from build123d import *

# Parameters (mm, degrees)
SKETCH4_R           = 2.5
BOSS_EXTRUDE1_DEPTH = 25
SKETCH5_R           = 2.5
CUT_EXTRUDE1_DEPTH  = 55.976783394
SKETCH6_R           = 3.25
CUT_EXTRUDE2_DEPTH  = 1
SKETCH7_R           = 2.5
CUT_EXTRUDE3_DEPTH  = 46.809522816
SKETCH8_R           = 3.25
CUT_EXTRUDE4_DEPTH  = 1


with BuildPart() as part:
    # Sketch4 → Boss-Extrude1 (new body)
    with BuildSketch(Plane(origin=(0, 0, 0), x_dir=(1, 0, 0), z_dir=(0, 1, 0))):
        with BuildLine():
            Line((12.859651739, 14.301163983), (32.859651739, 14.301163983))
            Line((32.859651739, 14.301163983), (32.859651739, 19.301163983))
            Line((32.859651739, 19.301163983), (12.859651739, 19.301163983))
            Line((12.859651739, 19.301163983), (12.859651739, 22.501163983))
            Line((12.859651739, 22.501163983), (3.559651739, 22.501163983))
            ThreePointArc((3.559651739, 22.501163983), (-3.511416073, 19.572231795), (-6.440348261, 12.501163983))
            Line((-6.440348261, 12.501163983), (-6.440348261, 3.001163983))
            Line((-6.440348261, 3.001163983), (-3.240348261, 3.001163983))
            Line((-3.240348261, 3.001163983), (-3.240348261, -16.998836017))
            Line((-3.240348261, -16.998836017), (1.759651739, -16.998836017))
            Line((1.759651739, -16.998836017), (1.759651739, 3.201163983))
            ThreePointArc((1.759651739, 3.201163983), (2.286859533, 4.473956189), (3.559651739, 5.001163983))
            ThreePointArc((3.559651739, 5.001163983), (8.862952598, 7.197863124), (11.059651739, 12.501163983))
            ThreePointArc((11.059651739, 12.501163983), (11.586859533, 13.773956189), (12.859651739, 14.301163983))
        make_face()
        with Locations(Location((3.559651739, 12.501163983, 0), (0, 0, 270))):
            Circle(SKETCH4_R, mode=Mode.SUBTRACT)
    extrude(amount=BOSS_EXTRUDE1_DEPTH)

    # Sketch5 → Cut-Extrude1 (cut, through all)
    with BuildSketch(Plane(origin=(0, 0, -19.301163983), x_dir=(-1, 0, 0), z_dir=(0, 0, -1))):
        with Locations((-22.859651739, 12.5)):
            Circle(SKETCH5_R)
    extrude(amount=-CUT_EXTRUDE1_DEPTH, mode=Mode.SUBTRACT)

    # Sketch6 → Cut-Extrude2 (cut)
    with BuildSketch(Plane.XY.offset(-14.301163983)):
        with Locations((22.859651739, 12.5)):
            Circle(SKETCH6_R)
    extrude(amount=-CUT_EXTRUDE2_DEPTH, mode=Mode.SUBTRACT)

    # Sketch7 → Cut-Extrude3 (cut, through all)
    with BuildSketch(Plane(origin=(1.759651739, 0, 0), x_dir=(0, 0, -1), z_dir=(1, 0, 0))):
        with Locations((-6.998836017, 12.5)):
            Circle(SKETCH7_R)
    extrude(amount=-CUT_EXTRUDE3_DEPTH, mode=Mode.SUBTRACT)

    # Sketch8 → Cut-Extrude4 (cut)
    with BuildSketch(Plane(origin=(1.759651739, 0, 0), x_dir=(0, 0, -1), z_dir=(1, 0, 0))):
        with Locations((-6.998836017, 12.5)):
            Circle(SKETCH8_R)
    extrude(amount=-CUT_EXTRUDE4_DEPTH, mode=Mode.SUBTRACT)


solid = part.part
Can you work these out from the model? Positions are in its coordinate system, mm. A direction names the side the tool comes from. Round coordinates to 2 decimals unless told otherwise and drop trailing zeros. Order: outer loops, then holes, each group sorted by start corner. A loop starts at its lowest first (then second) coordinate and runs counter-clockwise, first axis right, second up. Notation, with made-up numbers: (40, 43) -> (93, 43) arc R26 ccw to (93, 72) -> close; hole circle Ø11 at (-28, -21.75). An arc over 180 degrees is marked (long way). Write each question's results on one line, items separated by ' | '. Start each with the question number.
Item 1: If we section it at A-A, the plane y = 12.5: State how many separate pieces and enclosed holes the cut face has, then the cut area to 3 significant figures.
Item 2: If we section it at D-D, the plane x = 21: Write out the boundary of the cut face in (y, z).
Item 3: Which directions (+Z, -Z, +X, -X, +Y, -Y) give clear straight access to the entire face, cutting with the end or side of a thin tool? Please do faces 1 (the flat face through (24.9, 9.5, -14.301)), 2 (the flat face through (12.86, 12, -21)), 3 (the cylindrical face through (1.27, 15.24, 5.25)).
Item 4: Please list where these lines run through material, in increasing order: L1, parallel to X at y = 19.75, z = -1.5; L2, parallel to X at y = 10.75, z = -10.5; L3, parallel to Z at x = 14.5, y = 15.75.
Item 5: If we section it at C-C, the plane z = 7.5: Write out the boundary of the cut face in (x, y).
Item 6: Will these pins go through, and if not, where does the flat tip stop? pin 1 (8 mm diameter, centred on y = 12, z = -5, fed in from +X); pin 2 (1.5 mm diameter, centred on x = 17, y = 15.5, fed in from -Z); pin 3 (3 mm diameter, centred on y = 13.5, z = 8, fed in from +X); pin 4 (4 mm diameter, centred on x = 22.86, y = 12.5, fed in from +Z).
Item 7: If we section it at B-B, the plane y = 17: Write out the boundary of the cut face in (x, z).
Item 8: Thinking about a two-plate mould opening in Z: for faces 4 (the flat face through (24, 10, -15.301)), 5 (the cylindrical face through (4.311, 12.325, -10.117)), 6 (the flat face through (8, 12, -22.501)), which applies, +Z half, -Z half, draft (parallel to the pull), parting line (faces both ways), or undercut?
Results:
1) separate pieces: 3 | enclosed holes: 1 | area: 433 mm2
2) outline: (0, -19.3) -> (10.83, -19.3) -> (10.83, -15.3) -> (9.83, -15.3) -> (9.83, -14.3) -> (0, -14.3) -> close; (14.17, -19.3) -> (25, -19.3) -> (25, -14.3) -> (15.17, -14.3) -> (15.17, -15.3) -> (14.17, -15.3) -> close
3) face 1: +Z, +X, +Y, -Y | face 2: -Z, +X, +Y, -Y | face 3: +X
4) L1: x = -3.24 to 1.76 | L2: x = -6.44 to 2.06, 5.06 to 10.79 | L3: z = -19.3 to -14.3
5) outline: (-3.24, 0) -> (1.76, 0) -> (1.76, 9.29) -> (0.76, 9.29) -> (0.76, 10.05) -> (-3.24, 10.05) -> close; (-3.24, 14.95) -> (0.76, 14.95) -> (0.76, 15.71) -> (1.76, 15.71) -> (1.76, 25) -> (-3.24, 25) -> close
6) pin 1: stops at x = 10.19 | pin 2: stops at z = -19.3 | pin 3: stops at x = 0.76 | pin 4: passes through
7) outline: (-6.44, -12.5) arc R10 ccw to (3.56, -22.5) -> (12.86, -22.5) -> (12.86, -19.3) -> (32.86, -19.3) -> (32.86, -14.3) -> (12.86, -14.3) arc R1.8 cw to (11.06, -12.5) arc R7.5 ccw to (3.56, -5) arc R1.8 cw to (1.76, -3.2) -> (1.76, 17) -> (-3.24, 17) -> (-3.24, -3) -> (-6.44, -3) -> close; hole circle Ø5 at (3.56, -12.5)
8) face 4: +Z half | face 5: undercut | face 6: -Z half
